Check sheet for the modelled part. Datum: model origin and axes. Units: mm. A direction names the side the tool comes from. Round coordinates to 2 decimals unless told otherwise and drop trailing zeros. Write each loop counter-clockwise with the first axis right and the second up, starting at its lowest first coordinate (ties: lowest second). Pieces come first, ordered by that corner, then holes. Notation, with made-up numbers: (-20, -8.75) -> (36, -8.75) arc R13 ccw to (36, 12.25) -> close; hole circle Ø1 at (-4.75, 62). An arc over 180 degrees is marked (long way). One line per item, written item: value.
from build123d import *

# Parameters (mm, degrees)
BASE_FLANGE1_DEPTH = 50.8
SKETCH6_R          = 2.4892
CUT_EXTRUDE1_DEPTH = 87.054004212
SKETCH7_R          = 2.4892
CUT_EXTRUDE2_DEPTH = 87.054004212
FILLET1_R          = 3.175


# Sheet-metal steps are written as plain solids
with BuildPart() as part:
    # Sketch1 → Base-Flange1 (new, symmetric)
    with BuildSketch(Plane(origin=(0, 0, 0), x_dir=(1, 0, 0), z_dir=(0, 1, 0))):
        with BuildLine():
            Line((50.8, 0), (4.191, 0))
            ThreePointArc((4.191, 0), (1.22751548, -1.22751548), (0, -4.191))
            Line((0, -4.191), (0, -50.8))
            Line((0, -50.8), (3.429, -50.8))
            Line((3.429, -50.8), (3.429, -4.191))
            ThreePointArc((3.429, -4.191), (3.652184633, -3.652184633), (4.191, -3.429))
            Line((4.191, -3.429), (50.8, -3.429))
            Line((50.8, -3.429), (50.8, 0))
        make_face()
    extrude(amount=BASE_FLANGE1_DEPTH, both=True)

    # Sketch6 → Cut-Extrude1 (cut, through all)
    with BuildSketch(Plane(origin=(3.429, 0, 0), x_dir=(0, 0, -1), z_dir=(1, 0, 0))):
        with Locations((-38.1, 38.1)):
            Circle(SKETCH6_R)
        with Locations((-25.4, 38.1)):
            Circle(SKETCH6_R)
        with Locations((-38.1, 12.7)):
            Circle(SKETCH6_R)
        with Locations((-25.4, 12.7)):
            Circle(SKETCH6_R)
        with Locations((-38.1, -12.7)):
            Circle(SKETCH6_R)
        with Locations((-25.4, -12.7)):
            Circle(SKETCH6_R)
        with Locations((-38.1, -38.1)):
            Circle(SKETCH6_R)
        with Locations((-25.4, -38.1)):
            Circle(SKETCH6_R)
    extrude(amount=-CUT_EXTRUDE1_DEPTH, mode=Mode.SUBTRACT)

    # Sketch7 → Cut-Extrude2 (cut, through all)
    with BuildSketch(Plane.XY.offset(3.429)):
        with Locations((25.4, 38.1)):
            Circle(SKETCH7_R)
        with Locations((38.1, 38.1)):
            Circle(SKETCH7_R)
        with Locations((25.4, 12.7)):
            Circle(SKETCH7_R)
        with Locations((38.1, 12.7)):
            Circle(SKETCH7_R)
        with Locations((25.4, -12.7)):
            Circle(SKETCH7_R)
        with Locations((38.1, -12.7)):
            Circle(SKETCH7_R)
        with Locations((25.4, -38.1)):
            Circle(SKETCH7_R)
        with Locations((38.1, -38.1)):
            Circle(SKETCH7_R)
    extrude(amount=-CUT_EXTRUDE2_DEPTH, mode=Mode.SUBTRACT)

    # Fillet1
    fillet1_edges = [part.edges().sort_by_distance(p)[0] for p in [
        (1.7145, 50.8, 50.8),
        (1.7145, -50.8, 50.8),
        (50.8, 50.8, 1.7145),
        (50.8, -50.8, 1.7145),
    ]]
    fillet(fillet1_edges, radius=FILLET1_R)


solid = part.part
Item 1: Release check for a two-part mould opening along Y. For faces 1 (the cylindrical face through (35.613, -12.591, 1.739)), 2 (the cylindrical face through (26.74, 14.8, 1.74)), 3 (the flat face through (3, 50.8, 13)), 4 (the flat face through (50.8, 1, 2)) record: pulls with the +Y half, pulls with the -Y half, needs draft (parallel to the pull), parting line crosses it, or undercut.
Result set:
face 1: undercut
face 2: undercut
face 3: pulls with the +Y half
face 4: needs draft
Item 2: Sectioned sample at B-B (x = 38.1). Enter the section's corners in (y, z).
Result set:
outline: (-50.8, 0) -> (-40.59, 0) -> (-40.59, 3.43) -> (-50.8, 3.43) -> close; (-35.61, 0) -> (-15.19, 0) -> (-15.19, 3.43) -> (-35.61, 3.43) -> close; (-10.21, 0) -> (10.21, 0) -> (10.21, 3.43) -> (-10.21, 3.43) -> close; (15.19, 0) -> (35.61, 0) -> (35.61, 3.43) -> (15.19, 3.43) -> close; (40.59, 0) -> (50.8, 0) -> (50.8, 3.43) -> (40.59, 3.43) -> close
Item 3: Material ranges on line 1 along Y through (x, z) = (25.4, 0.9); line 2 along X through (y, z) = (12, 1); line 3 along Z through (x, y) = (39, 41), recorded low to high.
Result set:
line 1: -50.8 to -40.59, -35.61 to -15.19, -10.21 to 10.21, 15.19 to 35.61, 40.59 to 50.8
line 2: 1.47 to 23.01, 27.79 to 35.71, 40.49 to 50.8
line 3: 0 to 3.43
Item 4: Sectioned sample at C-C (y = -38.1). Enter the section's corners in (x, z).
Result set:
outline: (0, 4.19) arc R4.19 ccw to (4.19, 0) -> (22.91, 0) -> (22.91, 3.43) -> (4.19, 3.43) arc R0.76 cw to (3.43, 4.19) -> (3.43, 22.91) -> (0, 22.91) -> close; (0, 27.89) -> (3.43, 27.89) -> (3.43, 35.61) -> (0, 35.61) -> close; (0, 40.59) -> (3.43, 40.59) -> (3.43, 50.8) -> (0, 50.8) -> close; (27.89, 0) -> (35.61, 0) -> (35.61, 3.43) -> (27.89, 3.43) -> close; (40.59, 0) -> (50.8, 0) -> (50.8, 3.43) -> (40.59, 3.43) -> close
Item 5: Sectioned sample at D-D (z = 19). Enter the section's corners in (x, y), then the cut area to 3 significant figures.
Result set:
outline: (0, -50.8) -> (3.43, -50.8) -> (3.43, 50.8) -> (0, 50.8) -> close
area: 348 mm^2
Item 6: Tool access check on faces 5 (the flat face through (3.429, 1, 28)), 6 (the cylindrical face through (1.739, 35.892, 24.251)). Record the directions out of +Z, -Z, +X, -X, +Y, -Y that give a thin tool (end or side, any length) a straight path to the whole face; none if there is none.
Result set:
face 5: +Z, +X, +Y, -Y
face 6: +X, -X
Item 7: Sectioned sample at A-A (z = 38.1). Enter the section's corners in (x, y), then the cut area to 3 significant figures.
Result set:
outline: (0, -50.8) -> (3.43, -50.8) -> (3.43, -40.59) -> (0, -40.59) -> close; (0, -35.61) -> (3.43, -35.61) -> (3.43, -15.19) -> (0, -15.19) -> close; (0, -10.21) -> (3.43, -10.21) -> (3.43, 10.21) -> (0, 10.21) -> close; (0, 15.19) -> (3.43, 15.19) -> (3.43, 35.61) -> (0, 35.61) -> close; (0, 40.59) -> (3.43, 40.59) -> (3.43, 50.8) -> (0, 50.8) -> close
area: 280 mm^2
Item 8: Depth check by flat-ended pin: pin 1 (8 mm diameter, centred on y = 12.7, z = 38.1, fed in from +X); pin 2 (5.5 mm diameter, centred on x = 38.1, y = -38.1, fed in from -Z); pin 3 (6.5 mm diameter, centred on x = 25.4, y = -12.7, fed in from +Z); pin 4 (4 mm diameter, centred on y = -38.1, z = 38.1, fed in from +X). Enter the tip coordinate at first touch or a pass-through.
Result set:
pin 1: x = 3.43
pin 2: z = 0
pin 3: z = 3.43
pin 4: through
